from build123d import *

# Parameters (mm, degrees)
BOSS_EXTRU_1_DEPTH      = 180
ESQUISSE2_W             = 30
ESQUISSE2_H             = 6
ENL_V_MAT_EXTRU_1_DEPTH = 6


with BuildPart() as part:
    # Esquisse1 → Boss.-Extru.1 (new body)
    with BuildSketch(Plane.XY):
        with BuildLine():
            Line((0, 0), (9, 0))
            add(Edge.make_bspline(
                [(0, 18.154922759), (0.375552148, 8.111252363), (9, 0)],
                knots=[0.083456033, 0.083456033, 0.083456033, 1, 1, 1], degree=2))
            Line((0, 18.154922759), (0, 20))
            Line((0, 20), (-6, 20))
            Line((-6, 20), (-6, 0))
            Line((-6, 0), (0, 0))
        make_face()
    extrude(amount=BOSS_EXTRU_1_DEPTH)

    # Esquisse2 → Enlèv. mat.-Extru.1 (cut)
    with BuildSketch(Plane.ZY.offset(6)):
        with Locations((55, 3)):
            Rectangle(ESQUISSE2_W, ESQUISSE2_H)
        with Locations((125, 3)):
            Rectangle(ESQUISSE2_W, ESQUISSE2_H)
    extrude(amount=-ENL_V_MAT_EXTRU_1_DEPTH, mode=Mode.SUBTRACT)


solid = part.part
Verification items for the finished model (mm, model axes). A direction names the side the tool comes from. Coordinates: 2 decimals unless noted, no trailing zeros. Order: outer loops, then holes, each group sorted by start corner. A loop starts at its lowest first (then second) coordinate and runs counter-clockwise, first axis right, second up. Notation, with made-up numbers: (-8.5, 55.25) -> (32.5, 55.25) arc R12 cw to (32.5, 63.25) -> close; hole circle Ø10 at (51.5, 42.25). An arc over 180 degrees is marked (long way). Use CSV: the item, a comma, the result in double quotes. Start each with the question number.
Q1. Section check A-A, the plane x = -3.25. Record the cut outline in (y, z), and give its area (3 significant figures).
Q2. Depth check by flat-ended pin: P1, Ø8, axis at y = 18, z = 127, coming from the +X side; P2, Ø1.8, axis at x = -2, z = 58.5, coming from the -Y side; P3, Ø3, axis at y = 2, z = 121.5, coming from the -X side. Enter the tip coordinate at first touch or a pass-through.
Q3. Draft check along Z on faces 1 (the flat face through (-2, 8, 0)), 2 (the flat face through (-3, 3, 40)), 3 (the flat face through (-6, 10, 89)). Enter one of: +Z half, -Z half, draft (parallel to the pull), parting line (faces both ways), or undercut.
Q4. Tool access check on faces 4 (the flat face through (-2, 8, 180)), 5 (the flat face through (0, 3, 125)). Record the directions out of +Z, -Z, +X, -X, +Y, -Y that give a thin tool (end or side, any length) a straight path to the whole face; none if there is none.
Q5. Thickness scan on line 1 along X through (y, z) = (19, 40.5); line 2 along X through (y, z) = (12, 140.5); line 3 along Y through (x, z) = (3.5, 76). Record the ranges inside material, lowest first.
Returned:
1,outline,"(0, 0) -> (20, 0) -> (20, 180) -> (0, 180) -> (0, 140) -> (6, 140) -> (6, 110) -> (0, 110) -> (0, 70) -> (6, 70) -> (6, 40) -> (0, 40) -> close"
1,area,"3,240 mm^2"
2,P1,"stops at x = 0.53"
2,P2,"stops at y = 6"
2,P3,"stops at x = 0"
3,face 1,"-Z half"
3,face 2,"undercut"
3,face 3,"draft"
4,face 4,"+Z, +X, -X, +Y, -Y"
4,face 5,"-X, -Y"
5,line 1,"x = -6 to 0"
5,line 2,"x = -6 to 1.06"
5,line 3,"y = 0 to 6.67"
